from build123d import *

# Parameters (mm, degrees)
SKETCH1_R           = 10
BOSS_EXTRUDE1_DEPTH = 10.5
SKETCH3_R           = 17
BOSS_EXTRUDE2_DEPTH = 12
SKETCH4_R           = 1.55
CUT_EXTRUDE3_DEPTH  = 33.927951652
SKETCH5_R           = 1.55
CUT_EXTRUDE5_DEPTH  = 33.927951652
SKETCH6_R           = 1.75
CUT_EXTRUDE6_DEPTH  = 5.2
SKETCH7_R           = 1.75
CUT_EXTRUDE7_DEPTH  = 5.2


with BuildPart() as part:
    # Sketch1 → Boss-Extrude1 (new body)
    with BuildSketch(Plane.XY):
        with Locations(Location((0, 0, 0), (0, 0, 180))):
            Circle(SKETCH1_R)
    extrude(amount=BOSS_EXTRUDE1_DEPTH)

    # Sketch3 → Boss-Extrude2 (add)
    with BuildSketch(Plane.XY.offset(10.5)):
        Circle(SKETCH3_R)
    extrude(amount=BOSS_EXTRUDE2_DEPTH)

    # Sketch4 → Cut-Extrude3 (cut, through all)
    with BuildSketch(Plane.XY.offset(22.5)):
        with Locations((3, 0)):
            Circle(SKETCH4_R)
        with Locations((-3, 0)):
            Circle(SKETCH4_R)
    extrude(amount=-CUT_EXTRUDE3_DEPTH, mode=Mode.SUBTRACT)

    # Sketch5 → Cut-Extrude5 (cut, through all)
    with BuildSketch(Plane.XY.offset(22.5)):
        with Locations((13, 0)):
            Circle(SKETCH5_R)
        with Locations((0, -13)):
            Circle(SKETCH5_R)
        with Locations((-13, 0)):
            Circle(SKETCH5_R)
        with Locations((0, 13)):
            Circle(SKETCH5_R)
    extrude(amount=-CUT_EXTRUDE5_DEPTH, mode=Mode.SUBTRACT)

    # Sketch6 → Cut-Extrude6 (cut)
    with BuildSketch(Plane(origin=(0, 0, 10.5), x_dir=(-1, 0, 0), z_dir=(0, 0, -1))):
        with Locations((13, 0)):
            Circle(SKETCH6_R)
        with Locations((0, -13)):
            Circle(SKETCH6_R)
        with Locations((-13, 0)):
            Circle(SKETCH6_R)
        with Locations((0, 13)):
            Circle(SKETCH6_R)
    extrude(amount=-CUT_EXTRUDE6_DEPTH, mode=Mode.SUBTRACT)

    # Sketch7 → Cut-Extrude7 (cut)
    with BuildSketch(Plane.XY.offset(22.5)):
        with Locations((3, 0)):
            Circle(SKETCH7_R)
        with Locations((-3, 0)):
            Circle(SKETCH7_R)
    extrude(amount=-CUT_EXTRUDE7_DEPTH, mode=Mode.SUBTRACT)


solid = part.part
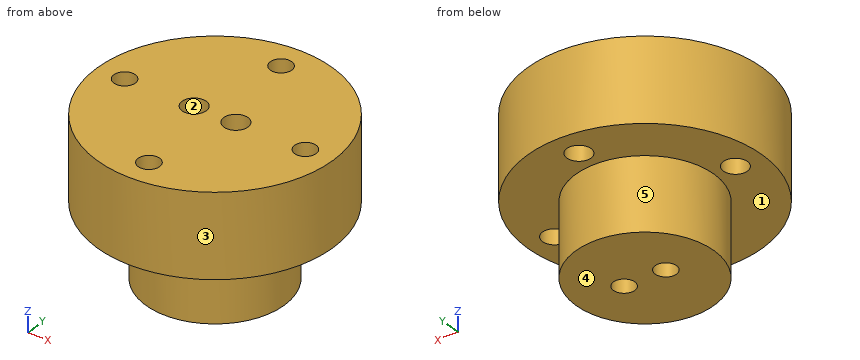
Could you check a few things on this model? Use its own coordinates, in mm. Face numbers are marked on the shaded views. A direction names the side the tool comes from. Give positions to 0.01 mm unless a question says otherwise; leave off trailing zeros. Order: outer loops, then holes, each group sorted by start corner. A loop starts at its lowest first (then second) coordinate and runs counter-clockwise, first axis right, second up. Notation, with made-up numbers: (42, 48) - (82, 48) arc R21 ccw to (82, 60) - close; hole circle Ø6 at (25, 8). An arc over 180 degrees is marked (long way). One line per item, written item: value. Start each with the question number.
1. Imagine slicing it at B-B on y = -13.5. List the corners of the cut face in (x, z) for me, plus the area to 3 significant figures.
2. If I drill on probe 1 along Y at (x, z) = (0, 12.95); probe 2 along X at (y, z) = (-1, 4.75); probe 3 along Z at (x, y) = (5.5, -10.5), over which ranges is the centre line in solid material (lowest first)?
3. Imagine slicing it at A-A on x = 0. List the corners of the cut face in (y, z) for me, plus the area to 3 significant figures.
4. Imagine slicing it at C-C on z = 8. List the corners of the cut face in (x, y) for me, plus the area to 3 significant figures.
5. For the marked faces 4 and 5, which set-ups out of +Z, -Z, +X, -X, +Y, -Y let a thin tool reach every point of the face, with its end or its side?
6. Imagine slicing it at D-D on x = 13. List the corners of the cut face in (y, z) for me, plus the area to 3 significant figures.
7. Thinking about a two-plate mould opening in X: for the marked faces 1, 2 and 3, which applies, +X half, -X half, draft (parallel to the pull), parting line (faces both ways), or undercut?
8. For P1, Ø4, axis at x = 0, y = 12.5, coming from the -Z side; P2, Ø12, axis at x = -10.5, z = 18, coming from the -Y side; P3, Ø5, axis at x = -13, z = 11, coming from the +Y side, each with a flat end and sliding along its axis, tell me the tip position at first contact or that it passes through.
Values:
1. outline: (-10.33, 10.5) - (-1.68, 10.5) - (-1.68, 15.7) - (-1.47, 15.7) - (-1.47, 22.5) - (-10.33, 22.5) - close; (1.47, 15.7) - (1.68, 15.7) - (1.68, 10.5) - (10.33, 10.5) - (10.33, 22.5) - (1.47, 22.5) - close
1. area: 211 mm²
2. probe 1: -17 to -14.75, -11.25 to 11.25, 14.75 to 17
2. probe 2: -9.95 to -4.18, -1.82 to 1.82, 4.18 to 9.95
2. probe 3: 10.5 to 22.5
3. outline: (-17, 10.5) - (-14.75, 10.5) - (-14.75, 15.7) - (-14.55, 15.7) - (-14.55, 22.5) - (-17, 22.5) - close; (-11.45, 15.7) - (-11.25, 15.7) - (-11.25, 10.5) - (-10, 10.5) - (-10, 0) - (10, 0) - (10, 10.5) - (11.25, 10.5) - (11.25, 15.7) - (11.45, 15.7) - (11.45, 22.5) - (-11.45, 22.5) - close; (14.55, 15.7) - (14.75, 15.7) - (14.75, 10.5) - (17, 10.5) - (17, 22.5) - (14.55, 22.5) - close
3. area: 539 mm²
4. outline: circle Ø20 at (0, 0); hole circle Ø3.1 at (-3, 0); hole circle Ø3.1 at (3, 0)
4. area: 299 mm²
5. face 4: -Z, +X, -X, +Y, -Y
5. face 5: -Z
6. outline: (-10.95, 10.5) - (-1.75, 10.5) - (-1.75, 15.7) - (-1.55, 15.7) - (-1.55, 22.5) - (-10.95, 22.5) - close; (1.55, 15.7) - (1.75, 15.7) - (1.75, 10.5) - (10.95, 10.5) - (10.95, 22.5) - (1.55, 22.5) - close
6. area: 224 mm²
7. face 1: draft
7. face 2: undercut
7. face 3: parting line
8. P1: z = 10.5
8. P2: y = -16.39
8. P3: y = 13.37
